Here's how the part is built. I have some questions about the finished solid (model axes, mm). A direction names the side the tool comes from. Give positions to 0.01 mm unless a question says otherwise; leave off trailing zeros. Write each loop counter-clockwise with the first axis right and the second up, starting at its lowest first coordinate (ties: lowest second). Pieces come first, ordered by that corner, then holes. Notation, with made-up numbers: (8, 58.5) -> (22, 58.5) arc R35 cw to (22, 94.5) -> close; hole circle Ø2 at (85.5, 1). An arc over 180 degrees is marked (long way). Use CSV: the item, a comma, the result in double quotes. Start each with the question number.
(1) Suppose I cut it at D-D on z = -7. List the corners of the cut face in (x, y) for me.
(2) I need wall thicknesses on L1, parallel to X at y = 9.5, z = 0; L2, parallel to X at y = 10.75, z = -0.75; L3, parallel to Z at x = 10, y = 16.5. Which ranges of each line are inside material? Lowest first, please. Write a range as [from, to].
(3) Which directions (+Z, -Z, +X, -X, +Y, -Y) give clear straight access to the entire face, cutting with the end or side of a thin tool? Please do faces 4 (the flat face through (8.77, 16.72, -9.24)), 5 (the flat face through (7, 16, 2)), 6 (the flat face through (-10, 15, -2)).
(4) Suppose I cut it at A-A on z = 0. List the corners of the cut face in (x, y) for me.
(5) Suppose I cut it at B-B on y = 11.75. List the corners of the cut face in (x, z) for me.
(6) Suppose I cut it at C-C on x = -10. List the corners of the cut face in (y, z) for me, plus the area to 3 significant figures.
(7) If we mould it in two halves opening along X, with no side actions, what happens to faces 1 (the flat face through (-8.841, 16.796, 9.24)), 2 (the flat face through (-20, 9, 0)), 3 (the flat face through (-0.3, 0.7, 9.2))? For each: pulls with the +X half, pulls with the -X half, needs draft (parallel to the pull), parting line crosses it, or undercut.
(8) For pin 1 Ø5 at (x, z) = (10, 0) entering from +Y; pin 2 Ø2.5 at (x, z) = (10, 0) entering from +Y, each with a flat end and sliding along its axis, tell me the tip position at first contact or that it passes through.
from build123d import *

# Parameters (mm, degrees)
SKETCH_1_W          = 40
SKETCH_1_H          = 20
SKETCH_1_R          = 1.6
EXTRUDE_1_DEPTH     = 20
CUT_EXTRUDE_1_DEPTH = 20
SKETCH_3_R          = 3.25
CUT_EXTRUDE_2_DEPTH = 5
CHAMFER_1_SIZE      = 1.5


with BuildPart() as part:
    # 草图1 → 凸台-拉伸1 (new body)
    with BuildSketch(Plane(origin=(0, 0, 0), x_dir=(1, 0, 0), z_dir=(0, 1, 0))):
        Rectangle(SKETCH_1_W, SKETCH_1_H)
        with Locations(Location((10, 0, 0), (0, 0, 270))):
            Circle(SKETCH_1_R, mode=Mode.SUBTRACT)
        with Locations(Location((-10, 0, 0), (0, 0, 90))):
            Circle(SKETCH_1_R, mode=Mode.SUBTRACT)
    extrude(amount=EXTRUDE_1_DEPTH)

    # 草图2 → 切除-拉伸1 (cut)
    with BuildSketch(Plane.XY.offset(10)):
        Polygon((-6, 15), (6, 15), (11, 20), (-11, 20), align=None)
    extrude(amount=-CUT_EXTRUDE_1_DEPTH, mode=Mode.SUBTRACT)

    # 草图3 → 切除-拉伸2 (cut)
    with BuildSketch(Plane(origin=(0, 20, 0), x_dir=(1, 0, 0), z_dir=(0, 1, 0))):
        with Locations(Location((10, 0, 0), (0, 0, 287.920213139))):
            Circle(SKETCH_3_R)
        with Locations(Location((-10, 0, 0), (0, 0, 252.079786861))):
            Circle(SKETCH_3_R)
    extrude(amount=-CUT_EXTRUDE_2_DEPTH, mode=Mode.SUBTRACT)

    # 倒角1
    chamfer_1_edges = [part.edges().sort_by_distance(p)[0] for p in [
        (-20, 20, 0),
        (-15.5, 20, 10),
        (15.5, 20, 10),
        (-15.5, 20, -10),
        (-8.5, 17.5, -10),
        (8.5, 17.5, -10),
        (0, 15, -10),
        (-8.5, 17.5, 10),
        (0, 15, 10),
        (8.5, 17.5, 10),
        (20, 20, 0),
        (0, 0, 10),
        (0, 0, -10),
        (20, 10, 10),
        (-20, 10, 10),
        (-20, 10, -10),
        (20, 10, -10),
        (15.5, 20, -10),
    ]]
    chamfer(chamfer_1_edges, length=CHAMFER_1_SIZE)


solid = part.part
Geometry says:
1,outline,"(-20, 0) -> (20, 0) -> (20, 18.5) -> (18.5, 20) -> (11, 20) -> (6, 15) -> (-6, 15) -> (-11, 20) -> (-18.5, 20) -> (-20, 18.5) -> close"
2,L1,"[-20, -11.6], [-8.4, 8.4], [11.6, 20]"
2,L2,"[-20, -11.41], [-8.59, 8.59], [11.41, 20]"
2,L3,"[-10, -3.25], [3.25, 10]"
3,face 4,"-Z, +Y"
3,face 5,"+Z, -Z, +Y"
3,face 6,"+Y"
4,outline,"(-20, 0) -> (-11.6, 0) -> (-11.6, 15) -> (-13.25, 15) -> (-13.25, 20) -> (-18.5, 20) -> (-20, 18.5) -> close; (-8.4, 0) -> (8.4, 0) -> (8.4, 15) -> (6.75, 15) -> (6.75, 15.75) -> (6, 15) -> (-6, 15) -> (-6.75, 15.75) -> (-6.75, 15) -> (-8.4, 15) -> close; (11.6, 0) -> (20, 0) -> (20, 18.5) -> (18.5, 20) -> (13.25, 20) -> (13.25, 15) -> (11.6, 15) -> close"
5,outline,"(-20, -8.5) -> (-18.5, -10) -> (18.5, -10) -> (20, -8.5) -> (20, 8.5) -> (18.5, 10) -> (-18.5, 10) -> (-20, 8.5) -> close; hole circle Ø3.2 at (-10, 0); hole circle Ø3.2 at (10, 0)"
6,outline,"(0, -8.5) -> (1.5, -10) -> (16.88, -10) -> (19, -8.5) -> (19, -3.25) -> (15, -3.25) -> (15, -1.6) -> (0, -1.6) -> close; (0, 1.6) -> (15, 1.6) -> (15, 3.25) -> (19, 3.25) -> (19, 8.5) -> (16.88, 10) -> (1.5, 10) -> (0, 8.5) -> close"
6,area,"301 mm²"
7,face 1,"undercut"
7,face 2,"pulls with the -X half"
7,face 3,"needs draft"
8,pin 1,"y = 15"
8,pin 2,"through"
